For this review, use the dimensioned drawing (mm, ordinates from the lowest corner) and the shaded views. Give positions to 0.01 mm unless a question says otherwise; leave off trailing zeros. Write each loop counter-clockwise with the first axis right and the second up, starting at its lowest first coordinate (ties: lowest second). Pieces come first, ordered by that corner, then holes. Notation, with made-up numbers: M -5.75,-37 L 13.25,-37 A27 ccw 13.25,-21 Z; hole C 20,0.5 d10. An arc over 180 degrees is marked long. Use a Markdown table: item, result. Add a question column.
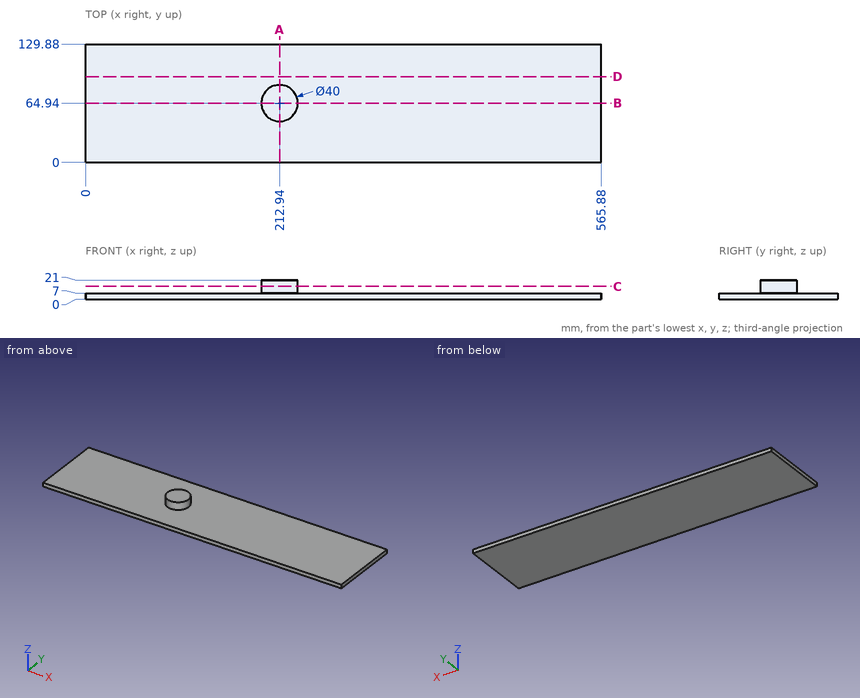
(1) For pin 1 (5 mm diameter, centred on x = 185, y = 106, fed in from +Z), flat-tipped, find the tip position at first contact; note if it passes through.
(2) Add section C-C on z = 14.5. Give the boundary of the cut face in (x, y).
(3) Wall thickness on L1, parallel to X at y = 63.5, z = 10.75; L2, parallel to Z at x = 85, y = 57; L3, parallel to X at y = 63, z = 19: over which ranges is each line inside the solid? List them lowest first.
(4) Add section A-A on x = 212.94. Give the boundary of the cut face in (y, z), then the cut area to 3 significant figures.
(5) Add section D-D on y = 94. Give the boundary of the cut face in (x, z), then the cut area to 3 significant figures.
(6) Add section B-B on y = 64.94. Give the boundary of the cut face in (x, z).
From the geometry:
| question | item | result |
|---|---|---|
| 1 | pin 1 | stops at z = 7 |
| 2 | outline | C 212.94,64.94 d40 |
| 3 | L1 | x = 192.99 to 232.89 |
| 3 | L2 | z = 0 to 7 |
| 3 | L3 | x = 193.03 to 232.85 |
| 4 | outline | M 0,0 L 129.88,0 L 129.88,7 L 84.94,7 L 84.94,21 L 44.94,21 L 44.94,7 L 0,7 Z |
| 4 | area | 1,470 mm^2 |
| 5 | outline | M 0,0 L 565.88,0 L 565.88,7 L 0,7 Z |
| 5 | area | 3,960 mm^2 |
| 6 | outline | M 0,0 L 565.88,0 L 565.88,7 L 232.94,7 L 232.94,21 L 192.94,21 L 192.94,7 L 0,7 Z |
